```python
from build123d import *

# Parameters (mm, degrees)
BOSS_EXTRUDE1_DEPTH = 0.12
FILLET1_R           = 3


with BuildPart() as part:
    # Sketch1 → Boss-Extrude1 (new, symmetric)
    with BuildSketch(Plane.XY):
        Polygon((0, 0), (1, 0), (4.909846718, -2.257351055), (7, -8), (7.652703645, -6.869484125), (5.725054187, -1.573310769), (1.267949192, 1), (0, 1), align=None)
    extrude(amount=BOSS_EXTRUDE1_DEPTH, both=True)

    # Fillet1
    # the kernel refuses this fillet: 3 mm, written as the material it adds along each edge
    with BuildSketch(Plane(origin=(1, 0, -0.12), x_dir=(-1, 0, 0), z_dir=(0, 0, 1))) as fillet1_piece_1:
        with BuildLine():
            CenterArc((FILLET1_R * 0.267949192431, FILLET1_R), FILLET1_R, 240, 30)
            Line((-FILLET1_R * 0.232050807569, FILLET1_R * 0.133974596216), (-FILLET1_R * 0.242050807569, FILLET1_R * 0.11665408814))
            Line((-FILLET1_R * 0.242050807569, FILLET1_R * 0.11665408814), (-FILLET1_R * 0.00535898384862, -FILLET1_R * 0.02))
            Line((-FILLET1_R * 0.00535898384862, -FILLET1_R * 0.02), (FILLET1_R * 0.267949192431, -FILLET1_R * 0.02))
            Line((FILLET1_R * 0.267949192431, -FILLET1_R * 0.02), (FILLET1_R * 0.267949192431, 0))
        make_face()
    extrude(amount=0.24)
    # the kernel refuses this fillet: 3 mm, written as the material it adds along each edge
    with BuildSketch(Plane(origin=(4.909846718, -2.257351055, -0.12), x_dir=(0.34202014332566544, -0.9396926207859095, 0), z_dir=(0, 0, 1))) as fillet1_2_piece_1:
        with BuildLine():
            CenterArc((FILLET1_R * 0.363970234266, -FILLET1_R), FILLET1_R, 90, 40)
            Line((-FILLET1_R * 0.27881737542, -FILLET1_R * 0.233955556881), (-FILLET1_R * 0.291673127614, -FILLET1_R * 0.218634668019))
            Line((-FILLET1_R * 0.291673127614, -FILLET1_R * 0.218634668019), (-FILLET1_R * 0.00727940468532, FILLET1_R * 0.02))
            Line((-FILLET1_R * 0.00727940468532, FILLET1_R * 0.02), (FILLET1_R * 0.363970234266, FILLET1_R * 0.02))
            Line((FILLET1_R * 0.363970234266, FILLET1_R * 0.02), (FILLET1_R * 0.363970234266, 0))
        make_face()
    extrude(amount=0.24)
    # the kernel refuses this fillet: 3 mm, written as the material it takes off along each edge
    with BuildSketch(Plane(origin=(1.267949192, 1, 2.129618943), x_dir=(-1, 0, 0), z_dir=(0, 0, -1))) as fillet1_3_piece_1:
        with BuildLine():
            CenterArc((FILLET1_R * 0.267949192431, -FILLET1_R), FILLET1_R, 90, 30)
            Line((-FILLET1_R * 0.232050807569, -FILLET1_R * 0.133974596216), (-FILLET1_R * 0.242050807569, -FILLET1_R * 0.11665408814))
            Line((-FILLET1_R * 0.242050807569, -FILLET1_R * 0.11665408814), (-FILLET1_R * 0.00535898384862, FILLET1_R * 0.02))
            Line((-FILLET1_R * 0.00535898384862, FILLET1_R * 0.02), (FILLET1_R * 0.267949192431, FILLET1_R * 0.02))
            Line((FILLET1_R * 0.267949192431, FILLET1_R * 0.02), (FILLET1_R * 0.267949192431, 0))
        make_face()
    extrude(amount=4.259237886, mode=Mode.SUBTRACT)
    # the kernel refuses this fillet: 3 mm, written as the material it takes off along each edge
    with BuildSketch(Plane(origin=(5.725054187, -1.573310769, -2.849776757), x_dir=(-0.8660254037844383, 0.5000000000000006, 0), z_dir=(0, 0, 1))) as fillet1_4_piece_1:
        with BuildLine():
            CenterArc((FILLET1_R * 0.363970234266, FILLET1_R), FILLET1_R, 230, 40)
            Line((-FILLET1_R * 0.27881737542, FILLET1_R * 0.233955556881), (-FILLET1_R * 0.291673127614, FILLET1_R * 0.218634668019))
            Line((-FILLET1_R * 0.291673127614, FILLET1_R * 0.218634668019), (-FILLET1_R * 0.00727940468532, -FILLET1_R * 0.02))
            Line((-FILLET1_R * 0.00727940468532, -FILLET1_R * 0.02), (FILLET1_R * 0.363970234266, -FILLET1_R * 0.02))
            Line((FILLET1_R * 0.363970234266, -FILLET1_R * 0.02), (FILLET1_R * 0.363970234266, 0))
        make_face()
    extrude(amount=5.699553514, mode=Mode.SUBTRACT)
    # the kernel refuses this fillet: 3 mm, written as the material it takes off along each edge
    with BuildSketch(Plane(origin=(7.652703645, -6.869484125, -3.612420866), x_dir=(-0.34202014332566655, 0.9396926207859092, 0), z_dir=(0, 0, 1))) as fillet1_5_piece_1:
        with BuildLine():
            CenterArc((1.396968346, 3), FILLET1_R, 221.810314896, 48.189685104)
            Line((-0.839099631, 1), (-0.883820991, 0.96))
            ThreePointArc((-0.883820991, 0.96), (-0.465512482, 0.461432743), (-0.045962667, -0.038567257))
            Line((-0.045962667, -0.038567257), (0, -0.06))
            Line((0, -0.06), (1.396968346, -0.06))
            Line((1.396968346, -0.06), (1.396968346, 0))
        make_face()
    extrude(amount=7.224841732, mode=Mode.SUBTRACT)


solid = part.part
```
Input: part model. Units: mm. Frame: model coordinates. Give positions to 0.01 mm unless a question says otherwise; leave off trailing zeros. Order: outer loops, then holes, each group sorted by start corner. A loop starts at its lowest first (then second) coordinate and runs counter-clockwise, first axis right, second up. Notation, with made-up numbers: (13, 39.25) - (62, 39.25) arc R32 cw to (62, 69.25) - close; hole circle Ø4 at (-1, 49.5). An arc over 180 degrees is marked (long way). Put each result on its own line as item: value.
Item 1: Ray query, L1, parallel to X at y = -5.25, z = 0.05; L2, parallel to X at y = -3, z = 0.05; L3, parallel to Y at x = 3.5, z = 0.05. Return the intervals inside material, ascending. Write a range as from..to.
Found:
L1: x = 6..7.06
L2: x = 5.16..6.24
L3: y = -1.44..-0.29
Item 2: Section query A-A, the plane z = 0.05. Return loops of the section in (x, y), then the cut area to 3 significant figures.
Found:
outline: (0, 0) - (0.2, 0) arc R3 cw to (1.7, -0.4) - (3.96, -1.71) arc R3 cw to (5.28, -3.28) - (7, -8) arc R3 ccw to (7.17, -5.56) - (6.1, -2.6) arc R3 ccw to (4.78, -1.03) - (1.96, 0.6) arc R3 ccw to (0.46, 1) - (0, 1) - close
area: 11.6 mm^2
Item 3: Section query B-B, the plane y = -6.75. Return loops of the section in (x, z), then the cut area to 3 significant figures.
Found:
outline: (6.55, -0.12) - (7.35, -0.12) - (7.35, 0.12) - (6.55, 0.12) - close
area: 0.193 mm^2
Item 4: Section query C-C, the plane x = 5. Return loops of the section in (y, z).
Found:
outline: (-2.71, -0.12) - (-1.17, -0.12) - (-1.17, 0.12) - (-2.71, 0.12) - close
